Job drawing, mm, ordinate dimensions from the low corner. One solid piece. A direction names the side the tool comes from. Coordinates: 2 decimals unless noted, no trailing zeros. Loops run counter-clockwise (first coordinate to the right, second up) from the corner with the lowest first, then second, coordinate; pieces in that order, holes last. Notation, with made-up numbers: (23.5, -28) - (39.5, -28) arc R13 ccw to (39.5, -20) - close; hole circle Ø11 at (56.5, 68). An arc over 180 degrees is marked (long way). Use a Markdown table: item, result. Add a question column.
1. Band-saw the part on A-A, the plane x = 12.7. Give the cut face in (y, z) (3 decimals).
2. 3-axis set-ups, long thin cutter, end or side, ignore diameter. For the marked faces 1 and 2: which of +Z, -Z, +X, -X, +Y, -Y reach the whole face in a straight line?
3. Wall check: probe 1 along Y at (x, z) = (12.7, 23.25); probe 2 along Y at (x, z) = (15, 8) (3 decimals). Give the ranges that are in metal, low to high. Write a range as [from, to].
4. Band-saw the part on B-B, the plane z = 12.7. Give the cut face in (x, y) (3 decimals).
5. Drop flat-ended pins along their axis: pin 1 (1 mm diameter, centred on x = 18, z = 9, fed in from +Y) (3 decimals); pin 2 (4 mm diameter, centred on x = 12.7, z = 12.7, fed in from -Y); pin 3 (11 mm diameter, centred on x = 6.5, y = 11.5, fed in from -Z) (3 decimals). Give the stop position or say it passes through.
6. Band-saw the part on C-C, the plane y = 12.7. Give the cut face in (x, z) (3 decimals).
7. Band-saw the part on D-D, the plane z = 23.5. Give the cut face in (x, y).
8. Pull direction X, two halves, no side cores. Call the marked faces 3 and 4: pulls with the +X half, pulls with the -X half, needs draft (parallel to the pull), parting line crosses it, or undercut.
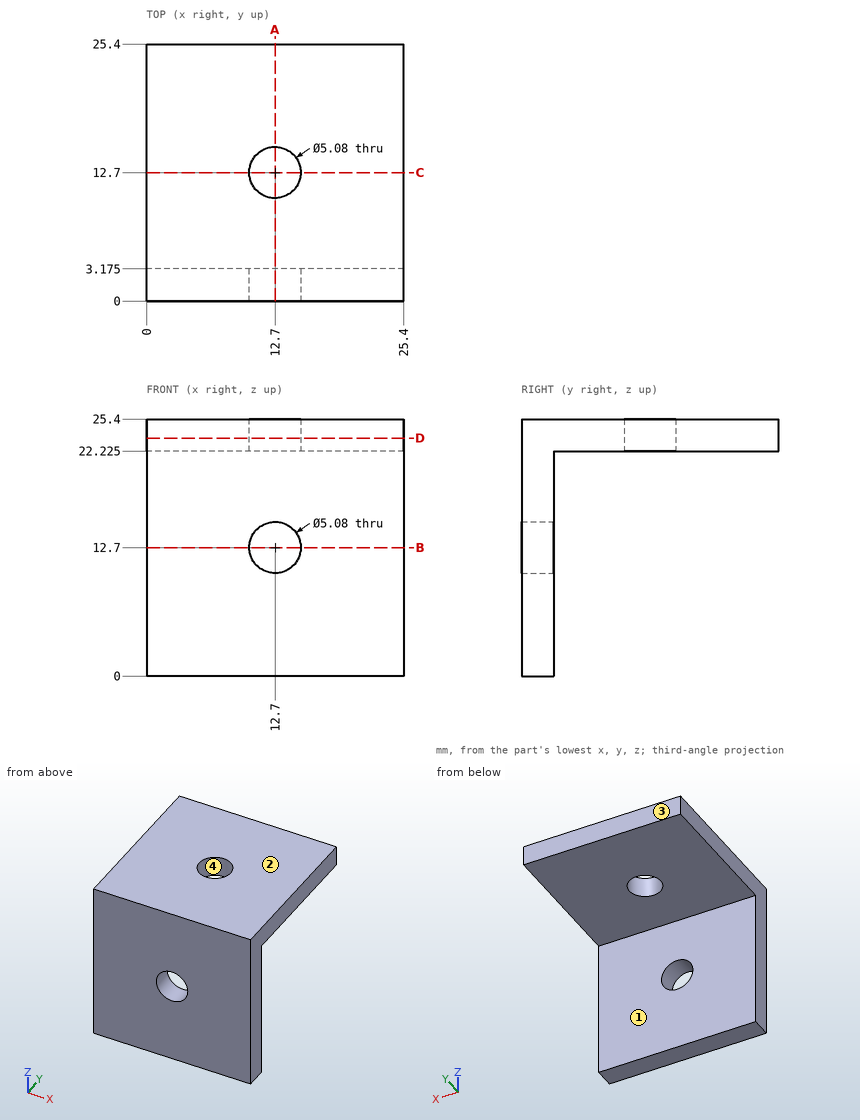
Geometry check:
| question | item | result |
|---|---|---|
| 1 | outline | (0, 0) - (3.175, 0) - (3.175, 10.16) - (0, 10.16) - close; (0, 15.24) - (3.175, 15.24) - (3.175, 22.225) - (10.16, 22.225) - (10.16, 25.4) - (0, 25.4) - close; (15.24, 22.225) - (25.4, 22.225) - (25.4, 25.4) - (15.24, 25.4) - close |
| 2 | face 1 | -Z, +X, -X, +Y |
| 2 | face 2 | +Z, +X, -X, +Y, -Y |
| 3 | probe 1 | y = [0, 10.16], [15.24, 25.4] |
| 3 | probe 2 | y = [0, 3.175] |
| 4 | outline | (0, 0) - (10.16, 0) - (10.16, 3.175) - (0, 3.175) - close; (15.24, 0) - (25.4, 0) - (25.4, 3.175) - (15.24, 3.175) - close |
| 5 | pin 1 | stops at y = 3.175 |
| 5 | pin 2 | passes through |
| 5 | pin 3 | stops at z = 22.225 |
| 6 | outline | (0, 22.225) - (10.16, 22.225) - (10.16, 25.4) - (0, 25.4) - close; (15.24, 22.225) - (25.4, 22.225) - (25.4, 25.4) - (15.24, 25.4) - close |
| 7 | outline | (0, 0) - (25.4, 0) - (25.4, 25.4) - (0, 25.4) - close; hole circle Ø5.08 at (12.7, 12.7) |
| 8 | face 3 | needs draft |
| 8 | face 4 | undercut |
